```python
from build123d import *

# Parameters (mm, degrees)
F3_W = 51.3915717602
F3_H = 13.7879867107


with BuildPart() as f1:
    # F0 (on Front) → F1 (revolve)
    with BuildSketch(Plane.XZ):
        Polygon((-456.6233754158, -12.6571897417), (-456.6233754158, -19.3570647389), (-335.4718983173, -19.3570647389), (-335.4718983173, 35.3837870061), (-349.2599129677, 35.3837870061), (-351.8936932087, 31.5794658113), (-351.8936932087, 25.0690672547), (-351.8936932087, 11.698897928), (-351.8936932087, -2.0408849232), (-367.9722547531, -2.0408849232), (-367.9722547531, -9.0839220211), (-417.7640676498, -9.0839220211), (-438.757032156, -12.6571897417), align=None)
    revolve(axis=Axis((-396.0476368666, 0, -19.3570647389), (1, 0, 0)))



with BuildPart() as f2:
    # F0 (on Front) → F2 (revolve)
    with BuildSketch(Plane.XZ):
        Polygon((-317.4982070923, -19.3570647389), (-212.301209569, -19.3570647389), (-212.301209569, -12.3819122091), (-250.7739365101, -12.3819122091), (-250.7739365101, -8.9349010959), (-285.9826683998, -8.9349010959), (-285.9826683998, -2.2870996036), (-301.4942109585, -2.2870996036), (-301.4942109585, 11.698897928), (-301.4942109585, 25.0690672547), (-301.4942109585, 31.4443483949), (-304.4488132, 35.1375713944), (-317.4982070923, 35.1375713944), align=None)
    revolve(axis=Axis((-264.8997083306, 0, -19.3570647389), (1, 0, 0)))


with BuildPart() as f1_1:
    add(f1.part)

    add(f2.part)  # F4 merges F2
    # F3 (on Front) → F4 (revolve)
    with BuildSketch(Plane.XZ):
        with Locations((-326.3935595751, 18.5928912833)):
            Rectangle(F3_W, F3_H)
    revolve(axis=Axis((-326.3935595751, 0, 11.698897928), (1, 0, 0)))


solid = f1_1.part
```
CAD build for the part. Positions are in the model's coordinates, mm. A direction names the side the tool comes from. Round coordinates to 2 decimals unless told otherwise and drop trailing zeros. Order: outer loops, then holes, each group sorted by start corner. A loop starts at its lowest first (then second) coordinate and runs counter-clockwise, first axis right, second up. Notation, with made-up numbers: (-21.5, 2.5) - (-9.5, 2.5) arc R35 cw to (-9.5, 37.5) - close; hole circle Ø4 at (-8.5, -31.5). An arc over 180 degrees is marked (long way). Answer as CSV lines item,"result". Start each with the question number.
1. Pin check, flat tips, straight feed: pin 1 (1.5 mm diameter, centred on x = -351, z = -56.5, fed in from +Y); pin 2 (4 mm diameter, centred on x = -300, z = 2.5, fed in from +Y); pin 3 (5 mm diameter, centred on y = 11, z = 19.5, fed in from +X); pin 4 (6.5 mm diameter, centred on y = -5, z = -14, fed in from +X). Stop position of each tip, or through.
2. Pull direction X, two halves, no side cores. Call faces 6 (the face through (-393.217, 3.935, -9.867)), 7 (the face through (-326.359, 8.39, 0.757)), 8 (the face through (-430.74, -2.422, -11.665)): +X half, -X half, draft (parallel to the pull), parting line (faces both ways), or undercut.
3. Saw through at B-B, the plane x = -297. Write the cut outline in (y, z), and give its area (3 significant figures).
4. Saw through at A-A, the plane x = -356. Write the cut outline in (y, z), and give its area (3 significant figures).
5. Drill centre lines: L1, parallel to X at y = -16, z = -66; L2, parallel to X at y = -1.5, z = -18; L3, parallel to Z at x = -377, y = 0. Where is each one in solid material? Low to high. Write a range as [from, to].
6. Tool access for faces 1 (the face through (-285.983, -8, -27)), 2 (the face through (-352.089, 0, 12)), 3 (the face through (-300.698, 0, 12)), 4 (the face through (-212.301, 0, -19)), 5 (the face through (-367.972, 7.5, -11.9)): list every direction of +Z, -Z, +X, -X, +Y, -Y with a clear straight run to the whole face (end or side of a thin tool).
Model answer:
1,pin 1,"stops at y = 38.41"
1,pin 2,"stops at y = 46.71"
1,pin 3,"stops at x = -300.7"
1,pin 4,"stops at x = -212.3"
2,face 6,"draft"
2,face 7,"undercut"
2,face 8,"-X half"
3,outline,"circle Ø34.14 at (0, -19.36)"
3,area,"915 mm²"
4,outline,"circle Ø34.63 at (0, -19.36)"
4,area,"942 mm²"
5,L1,"x = [-351.89, -335.47], [-317.5, -301.49]"
5,L2,"x = [-456.62, -335.47], [-317.5, -212.3]"
5,L3,"z = [-29.63, -9.08]"
6,face 1,"+X"
6,face 2,"+Z, -X, +Y, -Y"
6,face 3,"+Z, +X, +Y, -Y"
6,face 4,"+Z, -Z, +X, +Y, -Y"
6,face 5,"-X"
